For this review, take the finished solid that the model builds, in its own axes (mm). A direction names the side the tool comes from. Round coordinates to 2 decimals unless told otherwise and drop trailing zeros. Write each loop counter-clockwise with the first axis right and the second up, starting at its lowest first coordinate (ties: lowest second). Pieces come first, ordered by that corner, then holes. Notation, with made-up numbers: (22.25, -26) -> (80.25, -26) arc R14 cw to (80.25, -11) -> close; hole circle Ø2 at (20, -11.75). An arc over 180 degrees is marked (long way). Answer as CSV lines item,"result". Start each with the question number.
Item 1: Take a section at A-A on x = 5. Give the boundary of the cut face in (y, z).
Item 2: Wall thickness on probe 1 along Y at (x, z) = (-1.25, 86); probe 2 along Z at (x, y) = (-5.25, 213); probe 3 along Z at (x, y) = (13.25, 213): over which ranges is each line inside the solid? List them lowest first. Write a range as from..to.
Item 3: For pin 1 Ø10 at (x, y) = (13, 208) entering from +Z; pin 2 Ø3.5 at (y, z) = (225.33, 121.23) entering from -X; pin 3 Ø6 at (x, y) = (10, 215.5) entering from +Z, all flat-tipped, find the tip position at first contact; note any pin that passes through.
Item 4: Take a section at B-B on z = 78. Give the boundary of the cut face in (x, y), then the cut area to 3 significant figures.
Item 5: Take a section at C-C on x = 13.5. Give the boundary of the cut face in (y, z).
Item 6: Mouldability with a two-part tool opening along Y and no side actions: class faces 4 (the flat face through (4, 219, 71.227)), 5 (the conical face through (-5.6, 220.5, 115.4)), 6 (the cylindrical face through (14.334, 202.468, 116.334)) as +Y half, -Y half, draft (parallel to the pull), parting line (faces both ways), or undercut.
Item 7: Machinability: for faces 1 (the flat face through (4, 229.327, 90)), 2 (the flat face through (6, 204.327, 117)), 3 (the flat face through (-6, 209.327, 120)), which of the approach directions +Z, -Z, +X, -X, +Y, -Y give a long, thin tool a straight path to every point of the face, cutting with its end or side? Answer none if there is none.
```python
from build123d import *

# Parameters (mm, degrees)
SKETCH1_W                            = 48.407195654
SKETCH1_H                            = 28
BOSS_EXTRUDE1_DEPTH                  = 20
BOSS_EXTRUDE2_DEPTH                  = 3
CUT_EXTRUDE1_DEPTH                   = 20
CUT_EXTRUDE2_DEPTH                   = 266.217617444
F_6_0_6_DIAMETER_HOLE1_D             = 6
F_2_1_2_1_DIAMETER_HOLE1_D           = 2.1
F_2_1_2_1_DIAMETER_HOLE1_DEPTH       = 23
F_2_1_2_1_DIAMETER_HOLE1_CSINK_D     = 6.1
F_2_1_2_1_DIAMETER_HOLE1_CSINK_ANGLE = 90
FILLET1_R                            = 4


with BuildPart() as part:
    # Sketch1 → Boss-Extrude1 (new body)
    with BuildSketch(Plane(origin=(15.537250863, 0, 0), x_dir=(0, 0, -1), z_dir=(1, 0, 0))):
        with Locations((-95.430589359, 215.326974637)):
            Rectangle(SKETCH1_W, SKETCH1_H)
    extrude(amount=-BOSS_EXTRUDE1_DEPTH)

    # Sketch2 → Boss-Extrude2 (add)
    with BuildSketch(Plane.ZY.offset(4.462749137)):
        with BuildLine():
            Line((71.226991532, 201.326974637), (71.226991532, 229.326974637))
            Line((71.226991532, 229.326974637), (121.226991532, 229.326974637))
            ThreePointArc((121.226991532, 229.326974637), (131.226991532, 219.326974637), (121.226991532, 209.326974637))
            Line((121.226991532, 209.326974637), (119.634236905, 209.326974637))
            Line((119.634236905, 209.326974637), (119.634236905, 201.326974637))
            Line((119.634236905, 201.326974637), (71.226991532, 201.326974637))
        make_face()
    extrude(amount=BOSS_EXTRUDE2_DEPTH)

    # Sketch3 → Cut-Extrude1 (cut)
    with BuildSketch(Plane(origin=(15.537250863, 0, 0), x_dir=(0, 0, -1), z_dir=(1, 0, 0))):
        Polygon((-106.634187186, 211.932705929), (-106.634187186, 229.326974637), (-119.634187186, 229.326974637), (-119.634187186, 204.326974637), (-114.239918478, 204.326974637), align=None)
    extrude(amount=-CUT_EXTRUDE1_DEPTH, mode=Mode.SUBTRACT)

    # Sketch4 → Cut-Extrude2 (cut, through all)
    with BuildSketch(Plane.ZY.offset(7.462749137)):
        Polygon((71.226991532, 201.326974637), (111.468236905, 201.326974637), (103.468236905, 209.326974637), (71.226991532, 209.326974637), align=None)
    extrude(amount=-CUT_EXTRUDE2_DEPTH, mode=Mode.SUBTRACT)

    # Ø6.0 (6) Diameter Hole1 (through all)
    with Locations(Plane(origin=(-4.462749137, 0, 0), x_dir=(0, 0, -1), z_dir=(1, 0, 0))):
        with Locations((-121.226991532, 219.326974637)):
            Hole(F_6_0_6_DIAMETER_HOLE1_D / 2)

    # Ø2.1 (2.1) Diameter Hole1
    with Locations(Plane.ZY.offset(7.462749137)):
        with Locations((121.226991532, 225.326974637), (127.226991532, 219.326974637), (121.226991532, 213.326974637), (115.226991532, 219.326974637)):
            CounterSinkHole(F_2_1_2_1_DIAMETER_HOLE1_D / 2, F_2_1_2_1_DIAMETER_HOLE1_CSINK_D / 2, depth=F_2_1_2_1_DIAMETER_HOLE1_DEPTH, counter_sink_angle=F_2_1_2_1_DIAMETER_HOLE1_CSINK_ANGLE)

    # Fillet1
    fillet1_edges = [part.edges().sort_by_distance(p)[0] for p in [
        (15.537250863, 201.326974637, 115.551212045),
        (15.537250863, 209.326974637, 87.347614218),
        (15.537250863, 205.326974637, 107.468236905),
        (-7.462749137, 201.326974637, 115.551236905),
        (4.037250863, 201.326974637, 111.468236905),
        (-7.462749137, 205.326974637, 107.468236905),
        (-7.462749137, 209.326974637, 87.347614218),
        (4.037250863, 209.326974637, 103.468236905),
    ]]
    fillet(fillet1_edges, radius=FILLET1_R)


solid = part.part
```
Output values:
1,outline,"(201.33, 113.13) arc R4 ccw to (202.5, 110.3) -> (208.16, 104.64) arc R4 cw to (209.33, 101.81) -> (209.33, 71.23) -> (229.33, 71.23) -> (229.33, 106.63) -> (211.93, 106.63) -> (204.33, 114.24) -> (204.33, 119.63) -> (201.33, 119.63) -> close"
2,probe 1,"y = 209.33..229.33"
2,probe 2,"z = 71.23..120.23, 122.22..128.97"
2,probe 3,"z = 71.23..106.63"
3,pin 1,"stops at z = 119.63"
3,pin 2,"stops at x = -6.17"
3,pin 3,"stops at z = 106.63"
4,outline,"(-7.46, 213.33) arc R4 ccw to (-3.46, 209.33) -> (11.54, 209.33) arc R4 ccw to (15.54, 213.33) -> (15.54, 229.33) -> (-7.46, 229.33) -> close"
4,area,"453 mm^2"
5,outline,"(201.84, 113.13) arc R3.49 ccw to (202.86, 110.66) -> (208.52, 105) arc R4.51 cw to (209.84, 101.81) -> (209.84, 71.23) -> (229.33, 71.23) -> (229.33, 106.63) -> (211.93, 106.63) -> (204.33, 114.24) -> (204.33, 119.63) -> (201.84, 119.63) -> close"
6,face 4,"draft"
6,face 5,"undercut"
6,face 6,"-Y half"
7,face 1,"+Z, -Z, +X, -X, +Y"
7,face 2,"+Z, +X, +Y"
7,face 3,"+Z, +X, -X, -Y"
